Source: CAD feature listing. Evaluate the final solid. Frame: model axes, mm. A direction names the side the tool comes from. Give positions to 0.01 mm unless a question says otherwise; leave off trailing zeros. Order: outer loops, then holes, each group sorted by start corner. A loop starts at its lowest first (then second) coordinate and runs counter-clockwise, first axis right, second up. Notation, with made-up numbers: M 88.25,52 L 96.25,52 A25 ccw 96.25,81 Z; hole C 71,7.5 d7. An arc over 180 degrees is marked long. Use CSV: the item, a comma, the result in double quotes. Start each with the question number.
1. Section query B-B, the plane x = 6.25. Return the cut outline in (y, z), plus the area to 3 significant figures.
2. Line query: line 1 along X through (y, z) = (10.5, 0); line 2 along X through (y, z) = (13.5, 0); line 3 along Y through (x, z) = (2.75, -6). Output: solid intervals per line, ascending. Write a range as [from, to].
3. Section query A-A, the plane y = 8.25. Return the cut outline in (x, z), plus the area to 3 significant figures.
4. Reachability of faces 1 (the cylindrical face through (-1.802, 2.041, -5.723)), 2 (the cylindrical face through (4.3, 10.97, -2.24)), 3 (the flat face through (-3, 15.9, -2)) from +Z, -Z, +X, -X, +Y, -Y: full face, straight path, thin tool, end or side. Return the list, or none.
5. Pin query (flat end, axial travel): P1, Ø7, axis at x = -1, z = -1.5, coming from the +Y side; P2, Ø1.5, axis at y = 10, z = 0.5, coming from the -X side; P3, Ø5, axis at x = 5.5, y = -2, coming from the +Z side; P4, Ø3, axis at x = 5, y = 5.5, coming from the +Z side. Return the tip coordinate at first contact, or that it passes through.
6. Mould query, pull axis X, two halves, no side actions, for faces 4 (the flat face through (1, 4.2, 2)), 5 (the flat face through (5, 6.9, 2)), 6 (the cylindrical face through (4.3, 7.91, -2.24)), 7 (the cylindrical face through (-2.23, 9.97, 2.43)). Classes: released by +X, released by -X, zero draft, split by the parting line, or undercut.
from build123d import *


with BuildPart() as part:
    # Sketch1 → Revolve1 (revolve)
    with BuildSketch(Plane.XY, mode=Mode.PRIVATE) as revolve1_sk:
        with BuildLine():
            Line((4.079215611, -1.9), (5, -1.9))
            ThreePointArc((5, -1.9), (5.707106781, -1.607106781), (6, -0.9))
            Line((6, -0.9), (6, 4.9))
            Line((6, 4.9), (7, 4.9))
            Line((7, 4.9), (7, 6.9))
            Line((7, 6.9), (4.85, 6.9))
            Line((4.85, 6.9), (4.85, 8.9))
            ThreePointArc((4.85, 8.9), (5, 9.3), (4.85, 9.7))
            Line((4.85, 9.7), (4.85, 12.2))
            ThreePointArc((4.85, 12.2), (4.760969375, 12.873145601), (4.5, 13.5))
            Line((4.5, 13.5), (4.5, 15.9))
            Line((4.5, 15.9), (3.3, 15.9))
            Line((3.3, 15.9), (3.3, 4.2))
            Line((3.3, 4.2), (1.615549442, 4.2))
            ThreePointArc((1.615549442, 4.2), (0.821583836, 4.424364361), (0, 4.5))
            Line((0, 4.5), (0, 4.2))
            Line((0, 4.2), (0, -4.5))
            ThreePointArc((0, -4.5), (2.418677324, -3.794733192), (4.079215611, -1.9))
        make_face()
    revolve(revolve1_sk.sketch.rotate(Axis((0, 0, 0), (0, 1, 0)), 90), axis=Axis((0, 0, 0), (0, 1, 0)))


solid = part.part
Result set:
1,outline,"M 4.9,-3.15 L 6.9,-3.15 L 6.9,3.15 L 4.9,3.15 Z"
1,area,"12.6 mm2"
2,line 1,"[-4.85, -3.3], [3.3, 4.85]"
2,line 2,"[-4.5, -3.3], [3.3, 4.5]"
2,line 3,"[4.9, 6.9]"
3,outline,"C 0,0 d9.7; hole C 0,0 d6.6"
3,area,"39.7 mm2"
4,face 1,"-Y"
4,face 2,"+Y"
4,face 3,"+Z, -Z, +X, -X, +Y"
5,P1,"y = 15.9"
5,P2,"x = -5"
5,P3,"z = 5.07"
5,P4,"z = 6.06"
6,face 4,"undercut"
6,face 5,"zero draft"
6,face 6,"split by the parting line"
6,face 7,"undercut"
